```python
from build123d import *

# Parameters (mm, degrees)
SKETCH1_W                        = 350
SKETCH1_H                        = 132.2
SKETCH1_H_2                      = 25
BOSS_EXTRUDE1_DEPTH              = 15
CARRIAGEHOLES_D                  = 6
CARRIAGEHOLES_CBORE_D            = 10
CARRIAGEHOLES_CBORE_DEPTH        = 5
CARRIAGESETSCREWS_D              = 4.2
BOTTOMRAILHOLES_D                = 4.2
SKETCH10_W                       = 60
SKETCH10_H                       = 50
SKETCH10_H_2                     = 15
CUT_EXTRUDE1_DEPTH               = 4
SFUNUTHOLES_D                    = 6
SFUNUTHOLES_DEPTH                = 11
SFUNUTHOLES_CBORE_D              = 10
SFUNUTHOLES_CBORE_DEPTH          = 5
SFUNUTHOLES_TIP                  = 1.802581857
SKETCH13_W                       = 42
SKETCH13_H                       = 60
BKNOTCH_DEPTH                    = 6
M6X1_0_TAPPED_HOLE1_D            = 5
M6X1_0_TAPPED_HOLE1_DEPTH        = 15
M6X1_0_TAPPED_HOLE1_TIP          = 1.502151548
BFBLOCKHOLES_D                   = 5
BFBLOCKHOLES_DEPTH               = 11
SKETCH22_W                       = 60
SKETCH22_H                       = 51.1
CUT_EXTRUDE2_DEPTH               = 4
MOTORMOUNT_D                     = 5
CARRIAGEPLATESSCREWS_D           = 6.6
CARRIAGEPLATESSCREWS_CBORE_D     = 11.5
CARRIAGEPLATESSCREWS_CBORE_DEPTH = 7
M6X1_0_TAPPED_HOLE2_D            = 5


with BuildPart() as part:
    # Sketch1 → Boss-Extrude1 (new body)
    with BuildSketch(Plane.XY):
        with Locations((28.251813468, -4.511813374)):
            Rectangle(SKETCH1_W, SKETCH1_H)
        with Locations((28.251813468, 74.088186626)):
            Rectangle(SKETCH1_W, SKETCH1_H_2)
        with Locations((28.251813468, -83.111813374)):
            Rectangle(SKETCH1_W, SKETCH1_H_2)
    extrude(amount=BOSS_EXTRUDE1_DEPTH)

    # carriageHoles (through all)
    with Locations(Plane(origin=(37.718280998, 56.588186626, 15), x_dir=(1, 0, 0), z_dir=(0, 0, 1))):
        with Locations((0, 0), (0, -40), (-53, -40), (-53, 0), (0, -82.2), (0, -122.2), (-53, -122.2), (-53, -82.2), (-123.96646753, -82.2), (-123.96646753, -122.2), (-176.96646753, -122.2), (-176.96646753, -82.2), (-176.96646753, -40), (-123.96646753, -40), (-123.96646753, 0), (-176.96646753, 0)):
            CounterBoreHole(CARRIAGEHOLES_D / 2, CARRIAGEHOLES_CBORE_D / 2, CARRIAGEHOLES_CBORE_DEPTH)

    # carriageSetScrews (through all)
    with Locations(Plane(origin=(11.218280998, 36.588186626, 15), x_dir=(1, 0, 0), z_dir=(0, 0, 1))):
        with Locations((0, 0), (-123.96646753, -82.2), (-123.96646753, 0), (0, -82.2)):
            Hole(CARRIAGESETSCREWS_D / 2)

    # bottomRailHoles (through all)
    with Locations(Plane(origin=(-106.748186532, 76.569952861, 15), x_dir=(1, 0, 0), z_dir=(0, 0, 1))):
        with Locations((0, 0), (60, 0), (120, 0), (180, 0), (180, -162.16353247), (120, -162.16353247), (60, -162.16353247), (0, -162.16353247)):
            Hole(BOTTOMRAILHOLES_D / 2)

    # Sketch10 → Cut-Extrude1 (cut)
    with BuildSketch(Plane(origin=(0, 0, 0), x_dir=(-1, 0, 0), z_dir=(0, 0, -1))):
        with Locations((50.764952767, -4.511813374)):
            Rectangle(SKETCH10_W, SKETCH10_H)
        with Locations((50.764952767, -37.011813374)):
            Rectangle(SKETCH10_W, SKETCH10_H_2)
    extrude(amount=-CUT_EXTRUDE1_DEPTH, mode=Mode.SUBTRACT)

    # sfuNutHoles
    with Locations(Plane(origin=(-30.764952767, 7.488186626, 15), x_dir=(1, 0, 0), z_dir=(0, 0, 1))):
        with Locations((0, 0), (0, -24), (-40, -24), (-40, 0)):
            CounterBoreHole(SFUNUTHOLES_D / 2, SFUNUTHOLES_CBORE_D / 2, SFUNUTHOLES_CBORE_DEPTH, depth=SFUNUTHOLES_DEPTH)
            with Locations((0, 0, -(SFUNUTHOLES_DEPTH + SFUNUTHOLES_TIP / 2))):  # 118° drill point
                Cone(0, SFUNUTHOLES_D / 2, SFUNUTHOLES_TIP, mode=Mode.SUBTRACT)

    # Sketch13 → bkNotch (cut)
    with BuildSketch(Plane.XY.offset(15)):
        with Locations((182.251813468, -4.511813374)):
            Rectangle(SKETCH13_W, SKETCH13_H)
    extrude(amount=-BKNOTCH_DEPTH, mode=Mode.SUBTRACT)

    # M6x1.0 Tapped Hole1
    with Locations(Plane(origin=(187.161743151, 18.488186626, 9), x_dir=(1, 0, 0), z_dir=(0, 0, 1))):
        with Locations((0, 0), (-13, 0), (0, -46), (-13, -46)):
            Hole(M6X1_0_TAPPED_HOLE1_D / 2, depth=M6X1_0_TAPPED_HOLE1_DEPTH)
            with Locations((0, 0, -(M6X1_0_TAPPED_HOLE1_DEPTH + M6X1_0_TAPPED_HOLE1_TIP / 2))):  # 118° drill point
                Cone(0, M6X1_0_TAPPED_HOLE1_D / 2, M6X1_0_TAPPED_HOLE1_TIP, mode=Mode.SUBTRACT)

    # BFBlockHoles
    with Locations(Plane(origin=(-70.838256849, 18.488186626, 15), x_dir=(1, 0, 0), z_dir=(0, 0, 1))):
        with Locations((0, 0), (0, -46)):
            Hole(BFBLOCKHOLES_D / 2, depth=BFBLOCKHOLES_DEPTH)

    # Sketch22 → Cut-Extrude2 (cut)
    with BuildSketch(Plane(origin=(0, 0, 0), x_dir=(-1, 0, 0), z_dir=(0, 0, -1))):
        with Locations((50.764952767, -70.061813374)):
            Rectangle(SKETCH22_W, SKETCH22_H)
    extrude(amount=-CUT_EXTRUDE2_DEPTH, mode=Mode.SUBTRACT)

    # MotorMount (through all)
    with Locations(Plane(origin=(193.251813468, 32.733794894, 15), x_dir=(1, 0, 0), z_dir=(0, 0, 1))):
        with Locations((0, 0), (0, -74.991216537)):
            Hole(MOTORMOUNT_D / 2)

    # carriagePlatesScrews (through all)
    with Locations(Plane(origin=(11.218280998, 56.588186626, 15), x_dir=(1, 0, 0), z_dir=(0, 0, 1))):
        with Locations((0, 0), (0, -122.2), (-123.96646753, -122.2), (-123.96646753, 0)):
            CounterBoreHole(CARRIAGEPLATESSCREWS_D / 2, CARRIAGEPLATESSCREWS_CBORE_D / 2, CARRIAGEPLATESSCREWS_CBORE_DEPTH)

    # M6x1.0 Tapped Hole2 (through all)
    with Locations(Plane(origin=(134.678280998, -42.011813374, 0), x_dir=(-1, 0, 0), z_dir=(0, 0, -1))):
        with Locations((0, 0), (40, 37.5), (0, 75)):
            Hole(M6X1_0_TAPPED_HOLE2_D / 2)


solid = part.part
```
For this review, take the finished solid that the model builds, in its own axes (mm). A direction names the side the tool comes from. Round coordinates to 2 decimals unless told otherwise and drop trailing zeros. Order: outer loops, then holes, each group sorted by start corner. A loop starts at its lowest first (then second) coordinate and runs counter-clockwise, first axis right, second up.
Q1. Wall thickness on line 1 (X direction, y = 75.5, z = 7); line 2 (Y direction, x = 189, z = 1.25); line 3 (Y direction, x = -19.5, z = 13.75): over which ranges is each line inside the solid? List them lowest first.
Findings below:
line 1: x = -146.75 to -108.56, -104.94 to -48.56, -44.94 to 11.44, 15.06 to 71.44, 75.06 to 203.25
line 2: y = -95.61 to -29.21, -25.82 to 16.79, 20.18 to 86.59
line 3: y = -95.61 to -68.3, -62.93 to -28.3, -22.93 to 13.9, 19.27 to 53.9, 59.27 to 86.59
Q2. We need section B-B, the plane z = 12.25. State how many separate pieces and enclosed holes the cut face has, plus the area to 3 significant figures.
Findings below:
separate pieces: 1
enclosed holes: 43
area: 59,000 mm2
Q3. We need section A-A, the plane y = -54. Give the boundary of the cut face in (x, z).
Findings below:
outline: (-146.75, 0) - (-80.76, 0) - (-80.76, 4) - (-20.76, 4) - (-20.76, 0) - (203.25, 0) - (203.25, 15) - (-146.75, 15) - close
Q4. Machinability: for faces 1 (the flat face through (-13, 54, 10)), 2 (the cylindrical face through (-68.384, -18.337, 6.958)), which of the approach directions +Z, -Z, +X, -X, +Y, -Y give a long, thin tool a straight path to every point of the face, cutting with its end or side? Answer none if there is none.
Findings below:
face 1: +Z
face 2: +Z, -Z
Q5. Mouldability with a two-part tool opening along Y and no side actions: class faces 3 (the flat face through (-146.748, -3, 7)), 4 (the cylindrical face through (-86.899, 21.546, 12.535)), 5 (the flat face through (26, 86.588, 7)) as pulls with the +Y half, pulls with the -Y half, needs draft (parallel to the pull), parting line crosses it, or undercut.
Findings below:
face 3: needs draft
face 4: undercut
face 5: pulls with the +Y half
Q6. Insertion check: P1, Ø11, axis at x = -71.5, y = 5.5, coming from the +Z side; P2, Ø5.5, axis at x = 13, y = 57.5, coming from the +Z side; P3, Ø1.8, axis at y = -14, z = 11, coming from the +X side; P4, Ø4.5, axis at x = -56, z = 1.5, coming from the -Y side. Each pin has a flat end and moves straight along its axis. Give the tip position at first contact, or say it passes through.
Findings below:
P1: stops at z = 15
P2: stops at z = 8
P3: stops at x = 161.25
P4: stops at y = 20.49
